Here's how the part is built. I have some questions about the finished solid (model axes, mm). Face numbers are marked on the shaded views. A direction names the side the tool comes from. Round coordinates to 2 decimals unless told otherwise and drop trailing zeros. Loops run counter-clockwise (first coordinate to the right, second up) from the corner with the lowest first, then second, coordinate; pieces in that order, holes last. Notation, with made-up numbers: M 65,23.5 L 87,23.5 A16 ccw 87,33.5 Z; hole C 50.25,7.25 d5. An arc over 180 degrees is marked long. Use a Markdown table: item, result.
```python
from build123d import *

# Parameters (mm, degrees)
BOSS_EXTRUDE1_DEPTH     = 2
SKETCH1_4_W             = 84
SKETCH1_4_H             = 21
SKETCH1_4_W_2           = 80
SKETCH1_4_H_2           = 17
SKETCH1_4_W_3           = 6
SKETCH1_4_H_3           = 12
SKETCH1_4_H_4           = 4
BOSS_EXTRUDE2_DEPTH     = 11
SKETCH2_W               = 6
SKETCH2_H               = 3
SKETCH2_H_2             = 11
CUT_EXTRUDE1_DEPTH      = 9
SKETCH3_W               = 18
SKETCH3_H               = 9
CUT_EXTRUDE2_DEPTH      = 2
SKETCH4_W               = 4
SKETCH4_H               = 4
BOSS_EXTRUDE3_DEPTH     = 9
SKETCH6_R               = 0.5
SKETCH6_R_2             = 1.5
CUT_EXTRUDE3_DEPTH      = 1
CUT_EXTRUDE4_DEPTH      = 2
CUT_EXTRUDE5_DEPTH      = 34
CUT_EXTRUDE5_DEPTH_BACK = 13


with BuildPart() as part:
    # Sketch1 → Boss-Extrude1 (new body)
    with BuildSketch(Plane(origin=(0, 0, 0), x_dir=(1, 0, 0), z_dir=(0, 1, 0))):
        Polygon((-42, 10.5), (-42, -10.5), (42, -10.5), (42, 14.5), (62, 14.5), (62, 16.5), (40, 16.5), (36.380121198, 10.5), align=None)
    extrude(amount=BOSS_EXTRUDE1_DEPTH)

    # Sketch1_4 → Boss-Extrude2 (add)
    # profile 1 of 5: a face of its own
    with BuildSketch(Plane(origin=(0, 0, 0), x_dir=(1, 0, 0), z_dir=(0, 1, 0))):
        Polygon((36.380121198, 10.5), (42, 10.5), (42, 14.5), (62, 14.5), (62, 16.5), (40, 16.5), align=None)
    # profile 2 of 5: a face of its own
    with BuildSketch(Plane(origin=(0, 0, 0), x_dir=(1, 0, 0), z_dir=(0, 1, 0))):
        Rectangle(SKETCH1_4_W, SKETCH1_4_H)
        Rectangle(SKETCH1_4_W_2, SKETCH1_4_H_2, mode=Mode.SUBTRACT)
    # profile 3 of 5: a face of its own
    with BuildSketch(Plane(origin=(0, 0, 0), x_dir=(1, 0, 0), z_dir=(0, 1, 0))):
        Polygon((-14, -8.5), (-6, -8.5), (-6, 8.5), (-14, 8.5), (-14, 4.5), (-8, 4.5), (-8, 3.5), (-14, 3.5), align=None)
    # profile 4 of 5: a face of its own
    with BuildSketch(Plane(origin=(0, 0, 0), x_dir=(1, 0, 0), z_dir=(0, 1, 0))):
        with Locations((-37, -2.5)):
            Rectangle(SKETCH1_4_W_3, SKETCH1_4_H_3)
    # profile 5 of 5: a face of its own
    with BuildSketch(Plane(origin=(0, 0, 0), x_dir=(1, 0, 0), z_dir=(0, 1, 0))):
        with Locations((-37, 6.5)):
            Rectangle(SKETCH1_4_W_3, SKETCH1_4_H_4)
    extrude(amount=BOSS_EXTRUDE2_DEPTH)

    # Sketch2 → Cut-Extrude1 (cut)
    with BuildSketch(Plane(origin=(0, 11, 0), x_dir=(1, 0, 0), z_dir=(0, 1, 0))):
        with Locations((-37, 7)):
            Rectangle(SKETCH2_W, SKETCH2_H)
        with Locations((-37, -3)):
            Rectangle(SKETCH2_W, SKETCH2_H_2)
    extrude(amount=-CUT_EXTRUDE1_DEPTH, mode=Mode.SUBTRACT)

    # Sketch3 → Cut-Extrude2 (cut)
    with BuildSketch(Plane(origin=(0, 0, -10.5), x_dir=(-1, 0, 0), z_dir=(0, 0, -1))):
        with Locations((31, 6.5)):
            Rectangle(SKETCH3_W, SKETCH3_H)
    extrude(amount=-CUT_EXTRUDE2_DEPTH, mode=Mode.SUBTRACT)

    # Sketch4 → Boss-Extrude3 (add)
    with BuildSketch(Plane(origin=(0, 2, 0), x_dir=(1, 0, 0), z_dir=(0, 1, 0))):
        with Locations((0, 6.5)):
            Rectangle(SKETCH4_W, SKETCH4_H)
        with Locations((0, -6.5)):
            Rectangle(SKETCH4_W, SKETCH4_H)
        with Locations((34, 6.5)):
            Rectangle(SKETCH4_W, SKETCH4_H)
        with Locations((34, -6.5)):
            Rectangle(SKETCH4_W, SKETCH4_H)
    extrude(amount=BOSS_EXTRUDE3_DEPTH)

    # Sketch6 → Cut-Extrude3 (cut)
    # profile 1 of 2: a face of its own
    with BuildSketch(Plane(origin=(0, 0, -16.5), x_dir=(-1, 0, 0), z_dir=(0, 0, -1))):
        with BuildLine():
            ThreePointArc((-59.5, 5.5), (-60.085737838, 3.892019784), (-61.5684803, 3.037523452))
            Line((-61.5684803, 3.037523452), (-50.5, 4))
            ThreePointArc((-50.5, 4), (-52, 5.5), (-50.5, 7))
            Line((-50.5, 7), (-61.5684803, 7.962476548))
            ThreePointArc((-61.5684803, 7.962476548), (-60.085737838, 7.107980216), (-59.5, 5.5))
        make_face()
        with Locations((-55.5, 5.5)):
            Circle(SKETCH6_R, mode=Mode.SUBTRACT)
        with Locations((-53, 5.5)):
            Circle(SKETCH6_R, mode=Mode.SUBTRACT)
    # profile 2 of 2: a face of its own
    with BuildSketch(Plane(origin=(0, 0, -16.5), x_dir=(-1, 0, 0), z_dir=(0, 0, -1))):
        with Locations((-50.5, 5.5)):
            Circle(SKETCH6_R_2)
        with Locations((-50.5, 5.5)):
            Circle(SKETCH6_R, mode=Mode.SUBTRACT)
    extrude(amount=-CUT_EXTRUDE3_DEPTH, mode=Mode.SUBTRACT)

    # Sketch6_3 → Cut-Extrude4 (cut)
    with BuildSketch(Plane(origin=(0, 0, -16.5), x_dir=(-1, 0, 0), z_dir=(0, 0, -1))):
        with BuildLine():
            Line((-62, 8), (-62, 3))
            Line((-62, 3), (-61.5684803, 3.037523452))
            ThreePointArc((-61.5684803, 3.037523452), (-60.085737838, 3.892019784), (-59.5, 5.5))
            ThreePointArc((-59.5, 5.5), (-60.085737838, 7.107980216), (-61.5684803, 7.962476548))
            Line((-61.5684803, 7.962476548), (-62, 8))
        make_face()
    extrude(amount=-CUT_EXTRUDE4_DEPTH, mode=Mode.SUBTRACT)

    # Sketch7 → Cut-Extrude5 (cut, two sides: drawn at the far end of the back side and taken through both)
    with BuildSketch(Plane(origin=(42, 0, 0), x_dir=(0, 0, -1), z_dir=(1, 0, 0)).offset(-CUT_EXTRUDE5_DEPTH_BACK)):
        Polygon((10.5, 0), (16.5, 2), (16.5, 0), align=None)
        Polygon((10.5, 11), (16.5, 9), (16.5, 11), align=None)
    extrude(amount=CUT_EXTRUDE5_DEPTH + CUT_EXTRUDE5_DEPTH_BACK, mode=Mode.SUBTRACT)


solid = part.part
```
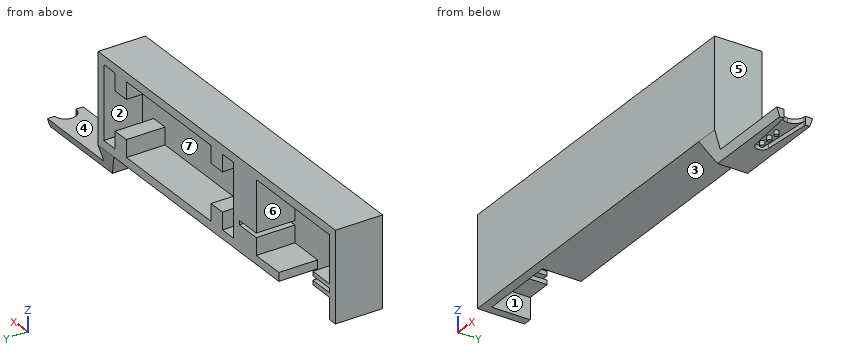
Q1. For the marked faces 1, 2 and 3, which set-ups out of +Z, -Z, +X, -X, +Y, -Y let a thin tool reach every point of the face, with its end or its side?
Return value:
| item | result |
|---|---|
| face 1 | -Z, +Y |
| face 2 | +Y |
| face 3 | -Z, -X, +Y, -Y |
Q2. Imagine slicing it at A-A, the plane x = 26. Please give me the cut outline in (y, z).
Return value:
| item | result |
|---|---|
| outline | M 0,-10.5 L 11,-10.5 L 11,-8.5 L 2,-8.5 L 2,8.5 L 11,8.5 L 11,10.5 L 0,10.5 Z |
Q3. We'd pull the mould along X, two halves only. Please class the marked faces 4, 5, 6 and 7: pulls with the +X half, pulls with the -X half, needs draft (parallel to the pull), parting line crosses it, or undercut.
Return value:
| item | result |
|---|---|
| face 4 | needs draft |
| face 5 | pulls with the +X half |
| face 6 | undercut |
| face 7 | undercut |
Q4. I need wall thicknesses on line 1 (X direction, y = 4.25, z = 1.75); line 2 (X direction, y = 9.5, z = 6.75); line 3 (Z direction, x = 30, y = 8). Which ranges of each line are inside material? Lowest first, please. Write a range as from..to.
Return value:
| item | result |
|---|---|
| line 1 | x = -42..-40, -14..-6, 40..42 |
| line 2 | x = -42..-40, -14..-6, -2..2, 32..36, 40..42 |
| line 3 | z = -10.5..-8.5, 8.5..10.5 |
Q5. Imagine slicing it at C-C, the plane z = -13. Please give me the cut outline in (x, y).
Return value:
| item | result |
|---|---|
| outline | M 37.89,0.83 L 42,0.83 L 42,10.17 L 37.89,10.17 Z |
Q6. Imagine slicing it at B-B, the plane z = -1.25. Please give me the cut outline in (x, y).
Return value:
| item | result |
|---|---|
| outline | M -42,0 L 42,0 L 42,11 L 40,11 L 40,2 L -6,2 L -6,11 L -14,11 L -14,2 L -40,2 L -40,11 L -42,11 Z |
Q7. Will these pins go through, and if not, where does the flat tip stop? P1, Ø2.5, axis at x = 21.5, y = 6, coming from the -Z side; P2, Ø8, axis at x = -29.5, z = -12.5, coming from the +Y side; P3, Ø2, axis at y = 6, z = 5.5, coming from the +X side; P4, Ø5, axis at x = 46, z = 2.5, coming from the +Y side.
Return value:
| item | result |
|---|---|
| P1 | stops at z = -10.5 |
| P2 | stops at y = 2 |
| P3 | stops at x = 42 |
| P4 | passes through |
